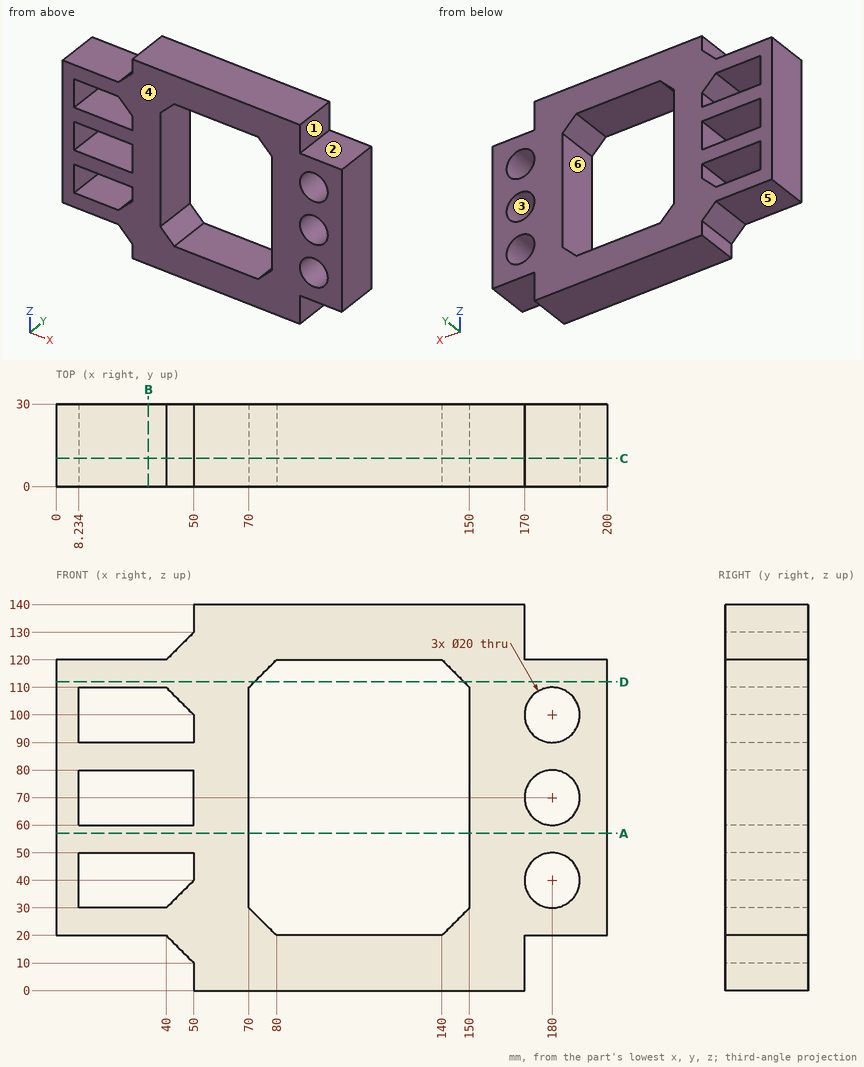
Print and shaded views of the part. All mm, measured from the part's lowest x, y and z. A direction names the side the tool comes from. Give positions to 0.01 mm unless a question says otherwise; leave off trailing zeros. Loops run counter-clockwise (first coordinate to the right, second up) from the corner with the lowest first, then second, coordinate; pieces in that order, holes last. Notation, with made-up numbers: (27, 37.25) -> (73, 37.25) arc R20 cw to (73, 57.25) -> close; hole circle Ø9 at (82, 77.5). An arc over 180 degrees is marked (long way). Use CSV: the item, a comma, the result in double quotes. Start each with the question number.
1) Slice it at B-B on x = 33.5. Give the cut face in (y, z), plus the area to 3 significant figures.
2) Slice it at C-C on y = 10.25. Give the number of separate pieces and of enclosed holes in the cut face, plus the area to 3 significant figures.
3) Wall check: line 1 (Z direction, x = 180, y = 17.5); line 2 (Z direction, x = 104, y = 18.5); line 3 (X direction, y = 19.75, z = 78). Give the ranges that are in metal, low to high.
4) Slice it at D-D on z = 112. Give the cut face in (x, y).
5) Slice it at A-A on z = 57. Give the cut face in (x, y).
6) Flat gauge pins, fed straight in: pin 1 Ø15 at (x, y) = (30.5, 13.5) entering from -Z; pin 2 Ø15 at (x, y) = (27.5, 13) entering from +Z; pin 3 Ø8 at (y, z) = (17.5, 134.5) entering from -X; pin 4 Ø16 at (x, z) = (180, 40) entering from -Y. Where does each tip first touch, or does it go through?
7) Tool access for the marked faces 4, 5 and 6: list every direction of +Z, -Z, +X, -X, +Y, -Y with a clear straight run to the whole face (end or side of a thin tool).
8) Mould opens along X. For the marked faces 1, 2 and 3 say: released by +X, released by -X, zero draft, split by the parting line, or undercut.
Computed values:
1,outline,"(0, 20) -> (30, 20) -> (30, 30) -> (0, 30) -> close; (0, 50) -> (30, 50) -> (30, 60) -> (0, 60) -> close; (0, 80) -> (30, 80) -> (30, 90) -> (0, 90) -> close; (0, 110) -> (30, 110) -> (30, 120) -> (0, 120) -> close"
1,area,"1,200 mm^2"
2,separate pieces,"1"
2,enclosed holes,"7"
2,area,"13,800 mm^2"
3,line 1,"z = 20 to 30, 50 to 60, 80 to 90, 110 to 120"
3,line 2,"z = 0 to 20, 120 to 140"
3,line 3,"x = 0 to 8.23, 50 to 70, 150 to 174, 186 to 200"
4,outline,"(0, 0) -> (72, 0) -> (72, 30) -> (0, 30) -> close; (148, 0) -> (200, 0) -> (200, 30) -> (148, 30) -> close"
5,outline,"(0, 0) -> (70, 0) -> (70, 30) -> (0, 30) -> close; (150, 0) -> (200, 0) -> (200, 30) -> (150, 30) -> close"
6,pin 1,"stops at z = 20"
6,pin 2,"stops at z = 120"
6,pin 3,"stops at x = 50"
6,pin 4,"passes through"
7,face 4,"+Z, -Z, +X, -X, -Y"
7,face 5,"-Z, -X, +Y, -Y"
7,face 6,"+Y, -Y"
8,face 1,"released by +X"
8,face 2,"zero draft"
8,face 3,"undercut"
